```python
from build123d import *

# Parameters (mm, degrees)
SKETCH_1_R          = 20
SKETCH_1_R_2        = 6.7
SKETCH_1_R_3        = 1.45
EXTRUDE_1_DEPTH     = 3
SKETCH_2_W          = 17.8
SKETCH_2_H          = 75
SKETCH_2_R          = 1.45
EXTRUDE_2_DEPTH     = 3
FILLET_1_R          = 15
SKETCH_3_R          = 3
CUT_EXTRUDE_1_DEPTH = 0.8


with BuildPart() as part:
    # 草图1 → 凸台-拉伸1 (new body)
    with BuildSketch(Plane.XY):
        Circle(SKETCH_1_R)
        Circle(SKETCH_1_R_2, mode=Mode.SUBTRACT)
        with Locations((0, 9.5)):
            Circle(SKETCH_1_R_3, mode=Mode.SUBTRACT)
        with Locations((8.227241336, 4.75)):
            Circle(SKETCH_1_R_3, mode=Mode.SUBTRACT)
        with Locations((8.227241336, -4.75)):
            Circle(SKETCH_1_R_3, mode=Mode.SUBTRACT)
        with Locations((0, -9.5)):
            Circle(SKETCH_1_R_3, mode=Mode.SUBTRACT)
        with Locations((-8.227241336, -4.75)):
            Circle(SKETCH_1_R_3, mode=Mode.SUBTRACT)
        with Locations((-8.227241336, 4.75)):
            Circle(SKETCH_1_R_3, mode=Mode.SUBTRACT)
    extrude(amount=EXTRUDE_1_DEPTH)

    # 草图2 → 凸台-拉伸2 (add)
    with BuildSketch(Plane.XY):
        with Locations((0, 50)):
            Rectangle(SKETCH_2_W, SKETCH_2_H)
        with Locations((0, 42.5)):
            Circle(SKETCH_2_R, mode=Mode.SUBTRACT)
        with Locations((0, 82.5)):
            Circle(SKETCH_2_R, mode=Mode.SUBTRACT)
    extrude(amount=EXTRUDE_2_DEPTH)

    # 圆角1
    fillet_1_edges = [part.edges().sort_by_distance(p)[0] for p in [
        (-8.9, 17.91061138, 1.5),
        (8.9, 17.91061138, 1.5),
    ]]
    fillet(fillet_1_edges, radius=FILLET_1_R)

    # 草图3 → 切除-拉伸1 (cut)
    with BuildSketch(Plane.XY.offset(3)):
        with Locations((0, 9.5)):
            Circle(SKETCH_3_R)
        with Locations((8.227241336, 4.75)):
            Circle(SKETCH_3_R)
        with Locations((8.227241336, -4.75)):
            Circle(SKETCH_3_R)
        with Locations((0, -9.5)):
            Circle(SKETCH_3_R)
        with Locations((-8.227241336, -4.75)):
            Circle(SKETCH_3_R)
        with Locations((-8.227241336, 4.75)):
            Circle(SKETCH_3_R)
    extrude(amount=-CUT_EXTRUDE_1_DEPTH, mode=Mode.SUBTRACT)


solid = part.part
```
Check sheet for the modelled part. Datum: model origin and axes. Units: mm. A direction names the side the tool comes from. Coordinates: 2 decimals unless noted, no trailing zeros. Write each loop counter-clockwise with the first axis right and the second up, starting at its lowest first coordinate (ties: lowest second). Pieces come first, ordered by that corner, then holes. Notation, with made-up numbers: M -37.5,13 L -29.5,13 A22 cw -29.5,50 Z; hole C 57.25,-12.5 d7. An arc over 180 degrees is marked long. Use one line per item in the form item = value.
Item 1: Gauge pin test, flat ends, axial feed: pin 1 Ø5.5 at (x, y) = (-8.23, -4.75) entering from +Z; pin 2 Ø1 at (y, z) = (69.5, 1) entering from -X; pin 3 Ø1.5 at (x, z) = (-11, 1) entering from +Y. Record the tip position at first contact, or that the pin passes through.
Answer below:
pin_1 = 2.2
pin_2 = -8.9
pin_3 = 19.35
Item 2: Sectioned sample at A-A, the plane y = 0. Record the cut outline in (x, z).
Answer below:
outline = M -20,0 L -6.7,0 L -6.7,3 L -20,3 Z; M 6.7,0 L 20,0 L 20,3 L 6.7,3 Z
Item 3: Release check for a two-part mould opening along Y. For faces 4 (the face through (-10.107, 19.675, 1.479)), 5 (the face through (10, 5, 2.2)), 6 (the face through (0, 23, 0)) record: pulls with the +Y half, pulls with the -Y half, needs draft (parallel to the pull), parting line crosses it, or undercut.
Answer below:
face_4 = pulls with the +Y half
face_5 = undercut
face_6 = needs draft
Item 4: Material ranges on L1, parallel to X at y = 38, z = 1.7; L2, parallel to X at y = -4.75, z = 2.85; L3, parallel to Y at x = -17.5, z = 1.2, recorded low to high. Write a range as from..to.
Answer below:
L1 = -8.9..8.9
L2 = -19.43..-11.23, -5.23..-4.73, 4.73..5.23, 11.23..19.43
L3 = -9.68..9.68
Item 5: Set-up check for faces 1 (the face through (1, -11, 2.2)), 2 (the face through (8.9, 56, 1)), 3 (the face through (-8.9, 56, 1)): record each of +Z, -Z, +X, -X, +Y, -Y from which the full face is reachable in a straight line by a thin tool's end or side.
Answer below:
face_1 = +Z
face_2 = +Z, -Z, +X, +Y
face_3 = +Z, -Z, -X, +Y
Item 6: Sectioned sample at C-C, the plane y = 42.5. Record the cut outline in (x, z).
Answer below:
outline = M -8.9,0 L -1.45,0 L -1.45,3 L -8.9,3 Z; M 1.45,0 L 8.9,0 L 8.9,3 L 1.45,3 Z
Item 7: Sectioned sample at D-D, the plane x = 16. Record the cut outline in (y, z).
Answer below:
outline = M -12,0 L 12,0 L 12,3 L -12,3 Z
Item 8: Sectioned sample at B-B, the plane z = 1.65. State how many separate pieces and enclosed holes the cut face has, and give its area (3 significant figures).
Answer below:
separate_pieces = 1
enclosed_holes = 9
area = 2,290 mm^2
